The model under review builds one solid part; all positions refer to its coordinate system, in mm. A direction names the side the tool comes from. Coordinates: 2 decimals unless noted, no trailing zeros. Order: outer loops, then holes, each group sorted by start corner. A loop starts at its lowest first (then second) coordinate and runs counter-clockwise, first axis right, second up. Notation, with made-up numbers: (11, -31) - (36, -31) arc R19 cw to (36, -20) - close; hole circle Ø11 at (55.25, 5). An arc over 180 degrees is marked (long way). Answer in a Markdown table with one row per item.
```python
from build123d import *

# Parameters (mm, degrees)
CUT_EXTRUDE2_REACH              = 84.5
M4_TAPPED_HOLE1_D               = 3.3
M4_TAPPED_HOLE1_DEPTH           = 10.1
M4_TAPPED_HOLE1_TIP             = 0.991420021
M4_TAPPED_HOLE1_ON_FACE_2_D     = 3.3
M4_TAPPED_HOLE1_ON_FACE_2_DEPTH = 10.1
M4_TAPPED_HOLE1_ON_FACE_2_TIP   = 0.991420021
M4_TAPPED_HOLE1_ON_FACE_3_D     = 3.3
M4_TAPPED_HOLE1_ON_FACE_3_DEPTH = 10.1
M4_TAPPED_HOLE1_ON_FACE_3_TIP   = 0.991420021
M4_TAPPED_HOLE1_ON_FACE_4_D     = 3.3
M4_TAPPED_HOLE1_ON_FACE_4_DEPTH = 10.1
M4_TAPPED_HOLE1_ON_FACE_4_TIP   = 0.991420021
CUT_EXTRUDE1_START              = -66.9
CUT_EXTRUDE1_DEPTH              = 66.9
M3_TAPPED_HOLE1_REACH           = 92.788
M3_TAPPED_HOLE1_BORE_R          = 1.25
F_2_4MM_DOWEL_HOLE1_D           = 2.38125
F_2_4MM_DOWEL_HOLE1_DEPTH       = 3
M4_CLEARANCE_HOLE2_D            = 4.3
M4_CLEARANCE_HOLE2_DEPTH        = 3


with BuildPart() as part:
    # Sketch1 → Revolve1 (revolve)
    with BuildSketch(Plane.XY, mode=Mode.PRIVATE) as revolve1_sk:
        Polygon((5.5, 66.9), (5.5, 0), (20, 0), (20, 3), (9.5, 3), (9.5, 36.5), (20, 36.5), (20, 77.5), (10, 77.5), (10, 100), (6, 100), (6, 66.9), align=None)
    revolve(revolve1_sk.sketch.rotate(Axis((0, 0, 0), (0, 1, 0)), 90), axis=Axis((0, 0, 0), (0, 1, 0)))

    # Sketch6 → Cut-Extrude2 (cut, up to next)
    with BuildSketch(Plane(origin=(0, 77.5, 0), x_dir=(1, 0, 0), z_dir=(0, 1, 0)), mode=Mode.PRIVATE) as cut_extrude2_sk1:
        with BuildLine():
            Line((-6.244997998, -19), (6.244997998, -19))
            ThreePointArc((6.244997998, -19), (0, -20), (-6.244997998, -19))
        make_face()
    cut_extrude2_tool1 = extrude(cut_extrude2_sk1.sketch, amount=-CUT_EXTRUDE2_REACH, mode=Mode.PRIVATE) & part.part
    add(cut_extrude2_tool1.solids().sort_by_distance((0, 77.5, 19.40087))[0], mode=Mode.SUBTRACT)

    # M4 Tapped Hole1
    with Locations(Plane(origin=(14.142135624, 67.5, -14.142135624), x_dir=(0.707106781187, 0, 0.707106781187), z_dir=(0.707106781187, 0, -0.707106781187))):
        with Locations((0, 0)):
            Hole(M4_TAPPED_HOLE1_D / 2, depth=M4_TAPPED_HOLE1_DEPTH)
            with Locations((0, 0, -(M4_TAPPED_HOLE1_DEPTH + M4_TAPPED_HOLE1_TIP / 2))):  # 118° drill point
                Cone(0, M4_TAPPED_HOLE1_D / 2, M4_TAPPED_HOLE1_TIP, mode=Mode.SUBTRACT)

    # M4 Tapped Hole1 on face 2
    with Locations(Plane(origin=(14.142135624, 46.5, -14.142135624), x_dir=(-0.707106781187, 0, -0.707106781187), z_dir=(0.707106781187, 0, -0.707106781187))):
        with Locations((0, 0)):
            Hole(M4_TAPPED_HOLE1_ON_FACE_2_D / 2, depth=M4_TAPPED_HOLE1_ON_FACE_2_DEPTH)
            with Locations((0, 0, -(M4_TAPPED_HOLE1_ON_FACE_2_DEPTH + M4_TAPPED_HOLE1_ON_FACE_2_TIP / 2))):  # 118° drill point
                Cone(0, M4_TAPPED_HOLE1_ON_FACE_2_D / 2, M4_TAPPED_HOLE1_ON_FACE_2_TIP, mode=Mode.SUBTRACT)

    # M4 Tapped Hole1 on face 3
    with Locations(Plane(origin=(-14.142135624, 46.5, -14.142135624), x_dir=(-0.707106781187, 0, 0.707106781187), z_dir=(-0.707106781187, 0, -0.707106781187))):
        with Locations((0, 0), (0, 21)):
            Hole(M4_TAPPED_HOLE1_ON_FACE_3_D / 2, depth=M4_TAPPED_HOLE1_ON_FACE_3_DEPTH)
            with Locations((0, 0, -(M4_TAPPED_HOLE1_ON_FACE_3_DEPTH + M4_TAPPED_HOLE1_ON_FACE_3_TIP / 2))):  # 118° drill point
                Cone(0, M4_TAPPED_HOLE1_ON_FACE_3_D / 2, M4_TAPPED_HOLE1_ON_FACE_3_TIP, mode=Mode.SUBTRACT)

    # M4 Tapped Hole1 on face 4
    with Locations(Plane(origin=(0, 67.5, 19), x_dir=(1, 0, 0), z_dir=(0, 0, 1))):
        with Locations((0, 0), (0, -21)):
            Hole(M4_TAPPED_HOLE1_ON_FACE_4_D / 2, depth=M4_TAPPED_HOLE1_ON_FACE_4_DEPTH)
            with Locations((0, 0, -(M4_TAPPED_HOLE1_ON_FACE_4_DEPTH + M4_TAPPED_HOLE1_ON_FACE_4_TIP / 2))):  # 118° drill point
                Cone(0, M4_TAPPED_HOLE1_ON_FACE_4_D / 2, M4_TAPPED_HOLE1_ON_FACE_4_TIP, mode=Mode.SUBTRACT)

    # Sketch3 → Cut-Extrude1 (cut)
    with BuildSketch(Plane.XZ.offset(CUT_EXTRUDE1_START)):
        with BuildLine():
            ThreePointArc((4.818762467, -2.651325759), (0, -5.885414894), (-4.818762467, -2.651325759))
            ThreePointArc((-4.818762467, -2.651325759), (0, 5.612925106), (4.818762467, -2.651325759))
        make_face()
    extrude(amount=CUT_EXTRUDE1_DEPTH, mode=Mode.SUBTRACT)

    # M3 Tapped Hole1 bore (on position points) → M3 Tapped Hole1 (cut, up to next)
    with BuildSketch(Plane(origin=(0, 16.5, 9.5), x_dir=(1, 0, 0), z_dir=(0, 0, 1)), mode=Mode.PRIVATE) as m3_tapped_hole1_sk1:
        Circle(M3_TAPPED_HOLE1_BORE_R)
    m3_tapped_hole1_tool1 = extrude(m3_tapped_hole1_sk1.sketch, amount=-M3_TAPPED_HOLE1_REACH, mode=Mode.PRIVATE) & part.part
    # M3 Tapped Hole1 bore (on position points) → M3 Tapped Hole1 (cut, up to next)
    with BuildSketch(Plane(origin=(0, 16.5, 9.5), x_dir=(1, 0, 0), z_dir=(0, 0, 1)), mode=Mode.PRIVATE) as m3_tapped_hole1_sk2:
        with Locations((0, 10)):
            Circle(M3_TAPPED_HOLE1_BORE_R)
    m3_tapped_hole1_tool2 = extrude(m3_tapped_hole1_sk2.sketch, amount=-M3_TAPPED_HOLE1_REACH, mode=Mode.PRIVATE) & part.part
    add(m3_tapped_hole1_tool1.solids().sort_by_distance((0, 16.5, 9.5))[0], mode=Mode.SUBTRACT)
    add(m3_tapped_hole1_tool2.solids().sort_by_distance((0, 26.5, 9.5))[0], mode=Mode.SUBTRACT)

    # Ø2.4mm Dowel Hole1
    with Locations(Plane(origin=(0, 0, 0), x_dir=(-1, 0, 0), z_dir=(0, -1, 0))):
        with Locations((0, -15.621), (0, 15.621)):
            Hole(F_2_4MM_DOWEL_HOLE1_D / 2, depth=F_2_4MM_DOWEL_HOLE1_DEPTH)

    # M4 Clearance Hole2
    with Locations(Plane(origin=(0, 3, 0), x_dir=(1, 0, 0), z_dir=(0, 1, 0))):
        with Locations((-10, -10), (0, 0), (-10, 10), (10, 10), (10, -10)):
            Hole(M4_CLEARANCE_HOLE2_D / 2, depth=M4_CLEARANCE_HOLE2_DEPTH)


solid = part.part
```
Item 1: We need section D-D, the plane y = 13. Write out the cut boundary in (x, z).
Check values:
| item | result |
|---|---|
| outline | circle Ø19 at (0, 0); hole (-4.82, -2.65) arc R5.21 ccw to (4.82, -2.65) arc R5.54 ccw (long way) to start |
Item 2: Clearance check with flat-ended pins moving along their axes: pin 1 Ø4 at (x, y) = (0, 26.5) entering from +Z; pin 2 Ø2 at (x, z) = (0, -15.621) entering from -Y; pin 3 Ø3.5 at (x, y) = (3, 64.5) entering from +Z; pin 4 Ø10 at (x, z) = (-14, 0) entering from -Y. State where each tip first meets the part, or that it passes through.
Check values:
| item | result |
|---|---|
| pin 1 | z = 9.5 |
| pin 2 | y = 36.5 |
| pin 3 | z = 19 |
| pin 4 | y = 0 |
Item 3: Tool access review of faces 1 (the face through (-0.27, 25.28, 7.51)), 2 (the face through (0.086, 33.918, -5.885)), 3 (the face through (0, 57, 19)), 4 (the face through (4, 3, -9)): name each direction out of +Z, -Z, +X, -X, +Y, -Y from which nothing blocks a thin tool from reaching the whole face with its end or side.
Check values:
| item | result |
|---|---|
| face 1 | +Z |
| face 2 | +Y, -Y |
| face 3 | +Z, +X, -X, +Y |
| face 4 | none |
Item 4: We need section A-A, the plane z = 0. Write out the cut boundary in (x, y).
Check values:
| item | result |
|---|---|
| outline | (-20, 0) - (-5.54, 0) - (-5.54, 66.9) - (-6, 66.9) - (-6, 100) - (-10, 100) - (-10, 77.5) - (-20, 77.5) - (-20, 36.5) - (-9.5, 36.5) - (-9.5, 3) - (-20, 3) - close; (5.54, 0) - (20, 0) - (20, 3) - (9.5, 3) - (9.5, 36.5) - (20, 36.5) - (20, 77.5) - (10, 77.5) - (10, 100) - (6, 100) - (6, 66.9) - (5.54, 66.9) - close |
Item 5: Mouldability with a two-part tool opening along Z and no side actions: class faces 5 (the face through (-2.854, 19.984, -9.061)), 6 (the face through (-0.04, 46.78, 8.08)), 7 (the face through (-5, 77.5, -9)), 8 (the face through (-3, 66.9, 5)) as +Z half, -Z half, draft (parallel to the pull), parting line (faces both ways), or undercut.
Check values:
| item | result |
|---|---|
| face 5 | parting line |
| face 6 | +Z half |
| face 7 | draft |
| face 8 | undercut |
Item 6: We need section B-B, the plane y = 74.5. Write out the cut boundary in (x, z) (3 decimals), then the cut area to 3 significant figures.
Check values:
| item | result |
|---|---|
| outline | (-6.245, 19) arc R20 ccw (long way) to (6.245, 19) - close; hole circle Ø12 at (0, 0) |
| area | 1,140 mm^2 |
Item 7: We need section C-C, the plane x = 11. State how many separate pieces and enclosed holes the cut face has, then the cut area to 3 significant figures.
Check values:
| item | result |
|---|---|
| separate pieces | 4 |
| enclosed holes | 2 |
| area | 1,420 mm^2 |
Item 8: To check wall thickness, follow line 1 (Y direction, x = -4.5, z = -11); line 2 (Y direction, x = 0, z = 15.5); line 3 (Y direction, x = -1, z = 13). State the ranges of each line that lie inside material, in increasing order. Write a range as from..to.
Check values:
| item | result |
|---|---|
| line 1 | 0..3, 36.5..77.5 |
| line 2 | 36.5..44.85, 48.15..65.85, 69.15..77.5 |
| line 3 | 0..3, 36.5..45.19, 47.81..66.19, 68.81..77.5 |
